from build123d import *

# Parameters (mm, degrees)
SKETCH1_R               = 35
BOSS_EXTRUDE1_DEPTH     = 10
CHAMFER1_SIZE           = 1
CUT_EXTRUDE1_DEPTH      = 11
SKETCH3_R               = 1.5
CUT_EXTRUDE2_DEPTH      = 11
CUT_EXTRUDE3_DEPTH      = 10
SKETCH5_R               = 9.729015648
BOSS_EXTRUDE2_DEPTH     = 3
SKETCH6_R               = 0.75
CUT_EXTRUDE4_DEPTH      = 36
CUT_EXTRUDE4_DEPTH_BACK = 36
CHAMFER2_SIZE           = 3


with BuildPart() as part:
    # Sketch1 → Boss-Extrude1 (new body)
    with BuildSketch(Plane(origin=(0, 0, 0), x_dir=(0, 0, -1), z_dir=(1, 0, 0))):
        Circle(SKETCH1_R)
        with BuildLine():
            Line((-5, 29.580398915), (-5, 8.660254038))
            ThreePointArc((-5, 8.660254038), (0, -10), (5, 8.660254038))
            Line((5, 8.660254038), (5, 29.580398915))
            ThreePointArc((5, 29.580398915), (0, -30), (-5, 29.580398915))
        make_face(mode=Mode.SUBTRACT)
    extrude(amount=BOSS_EXTRUDE1_DEPTH)

    # Chamfer1
    chamfer1_edges = [part.edges().sort_by_distance(p)[0] for p in [
        (0, 0, 35),
        (10, 0, 35),
    ]]
    chamfer(chamfer1_edges, length=CHAMFER1_SIZE)

    # Sketch2 → Cut-Extrude1 (cut, through all)
    with BuildSketch(Plane(origin=(10, 0, 0), x_dir=(0, 0, -1), z_dir=(1, 0, 0))):
        with BuildLine():
            Line((0, 35), (0, 34))
            ThreePointArc((0, 34), (3.553967751, 33.813744443), (7.068997488, 33.257018425))
            Line((7.068997488, 33.257018425), (7.276909179, 34.235166026))
            ThreePointArc((7.276909179, 34.235166026), (3.658496214, 34.808266338), (0, 35))
        make_face()
        with BuildLine():
            Line((15.185930869, 31.533910377), (14.75204713, 30.632941509))
            ThreePointArc((14.75204713, 30.632941509), (17.873248174, 28.923122233), (20.79862617, 26.896415178))
            Line((20.79862617, 26.896415178), (21.410350469, 27.687486213))
            ThreePointArc((21.410350469, 27.687486213), (18.398931943, 29.773802299), (15.185930869, 31.533910377))
        make_face()
        with BuildLine():
            Line((27.364101886, 21.822143065), (26.582270404, 21.198653263))
            ThreePointArc((26.582270404, 21.198653263), (28.652512594, 18.303920947), (30.408831861, 15.208647043))
            Line((30.408831861, 15.208647043), (31.303209268, 15.655960191))
            ThreePointArc((31.303209268, 15.655960191), (29.495233553, 18.842271563), (27.364101886, 21.822143065))
        make_face()
        with BuildLine():
            Line((34.122476926, 7.788232688), (33.147549014, 7.565711755))
            ThreePointArc((33.147549014, 7.565711755), (33.756795496, 4.059403634), (33.996195462, 0.508619839))
            Line((33.996195462, 0.508619839), (34.996083563, 0.523579246))
            ThreePointArc((34.996083563, 0.523579246), (34.749642422, 4.178797859), (34.122476926, 7.788232688))
        make_face()
        with BuildLine():
            Line((34.122476926, -7.788232688), (33.147549014, -7.565711755))
            ThreePointArc((33.147549014, -7.565711755), (32.175131049, -10.989128353), (30.850195615, -14.292145763))
            Line((30.850195615, -14.292145763), (31.75755431, -14.712502991))
            ThreePointArc((31.75755431, -14.712502991), (33.121458433, -11.312338011), (34.122476926, -7.788232688))
        make_face()
        with BuildLine():
            Line((27.364101886, -21.822143065), (26.582270404, -21.198653263))
            ThreePointArc((26.582270404, -21.198653263), (24.220787296, -23.861128698), (21.593936175, -26.262176614))
            Line((21.593936175, -26.262176614), (22.229051944, -27.034593573))
            ThreePointArc((22.229051944, -27.034593573), (24.933163393, -24.562926601), (27.364101886, -21.822143065))
        make_face()
        with BuildLine():
            Line((15.185930869, -31.533910377), (14.75204713, -30.632941509))
            ThreePointArc((14.75204713, -30.632941509), (11.469219571, -32.007139866), (8.060732842, -33.030661302))
            Line((8.060732842, -33.030661302), (8.29781322, -34.00215134))
            ThreePointArc((8.29781322, -34.00215134), (11.806549558, -32.948526333), (15.185930869, -31.533910377))
        make_face()
        with BuildLine():
            Line((0, -35), (0, -34))
            ThreePointArc((0, -34), (-3.553967751, -33.813744443), (-7.068997488, -33.257018425))
            Line((-7.068997488, -33.257018425), (-7.276909179, -34.235166026))
            ThreePointArc((-7.276909179, -34.235166026), (-3.658496214, -34.808266338), (0, -35))
        make_face()
        with BuildLine():
            Line((-15.185930869, -31.533910377), (-14.75204713, -30.632941509))
            ThreePointArc((-14.75204713, -30.632941509), (-17.873248174, -28.923122233), (-20.79862617, -26.896415178))
            Line((-20.79862617, -26.896415178), (-21.410350469, -27.687486213))
            ThreePointArc((-21.410350469, -27.687486213), (-18.398931943, -29.773802299), (-15.185930869, -31.533910377))
        make_face()
        with BuildLine():
            Line((-27.364101886, -21.822143065), (-26.582270404, -21.198653263))
            ThreePointArc((-26.582270404, -21.198653263), (-28.652512594, -18.303920947), (-30.408831861, -15.208647043))
            Line((-30.408831861, -15.208647043), (-31.303209268, -15.655960191))
            ThreePointArc((-31.303209268, -15.655960191), (-29.495233553, -18.842271563), (-27.364101886, -21.822143065))
        make_face()
        with BuildLine():
            Line((-34.122476926, -7.788232688), (-33.147549014, -7.565711755))
            ThreePointArc((-33.147549014, -7.565711755), (-33.756795496, -4.059403634), (-33.996195462, -0.508619839))
            Line((-33.996195462, -0.508619839), (-34.996083563, -0.523579246))
            ThreePointArc((-34.996083563, -0.523579246), (-34.749642422, -4.178797859), (-34.122476926, -7.788232688))
        make_face()
        with BuildLine():
            Line((-34.122476926, 7.788232688), (-33.147549014, 7.565711755))
            ThreePointArc((-33.147549014, 7.565711755), (-32.175131049, 10.989128353), (-30.850195615, 14.292145763))
            Line((-30.850195615, 14.292145763), (-31.75755431, 14.712502991))
            ThreePointArc((-31.75755431, 14.712502991), (-33.121458433, 11.312338011), (-34.122476926, 7.788232688))
        make_face()
        with BuildLine():
            Line((-27.364101886, 21.822143065), (-26.582270404, 21.198653263))
            ThreePointArc((-26.582270404, 21.198653263), (-24.220787296, 23.861128698), (-21.593936175, 26.262176614))
            Line((-21.593936175, 26.262176614), (-22.229051944, 27.034593573))
            ThreePointArc((-22.229051944, 27.034593573), (-24.933163393, 24.562926601), (-27.364101886, 21.822143065))
        make_face()
        with BuildLine():
            Line((-15.185930869, 31.533910377), (-14.75204713, 30.632941509))
            ThreePointArc((-14.75204713, 30.632941509), (-11.469219571, 32.007139866), (-8.060732842, 33.030661302))
            Line((-8.060732842, 33.030661302), (-8.29781322, 34.00215134))
            ThreePointArc((-8.29781322, 34.00215134), (-11.806549558, 32.948526333), (-15.185930869, 31.533910377))
        make_face()
    extrude(amount=-CUT_EXTRUDE1_DEPTH, mode=Mode.SUBTRACT)

    # Sketch3 → Cut-Extrude2 (cut, through all)
    with BuildSketch(Plane.ZY):
        Circle(SKETCH3_R)
    extrude(amount=-CUT_EXTRUDE2_DEPTH, mode=Mode.SUBTRACT)

    # Sketch4 → Cut-Extrude3 (cut)
    with BuildSketch(Plane.ZY):
        with BuildLine():
            Line((-3.865553001, -2.4), (3.865553001, -2.4))
            ThreePointArc((3.865553001, -2.4), (4.55, 0), (3.865553001, 2.4))
            Line((3.865553001, 2.4), (-3.865553001, 2.4))
            ThreePointArc((-3.865553001, 2.4), (-4.55, 0), (-3.865553001, -2.4))
        make_face()
    extrude(amount=-CUT_EXTRUDE3_DEPTH, mode=Mode.SUBTRACT)

    # Sketch5 → Boss-Extrude2 (add)
    with BuildSketch(Plane.ZY):
        Circle(SKETCH5_R)
        with BuildLine():
            Line((-3.865553001, 2.4), (3.865553001, 2.4))
            ThreePointArc((3.865553001, 2.4), (4.568220616, 0), (3.865553001, -2.4))
            Line((3.865553001, -2.4), (-3.865553001, -2.4))
            ThreePointArc((-3.865553001, -2.4), (-4.568220616, 0), (-3.865553001, 2.4))
        make_face(mode=Mode.SUBTRACT)
    extrude(amount=BOSS_EXTRUDE2_DEPTH)

    # Sketch6 → Cut-Extrude4 (cut, two sides)
    with BuildSketch(Plane(origin=(0, 0, 0), x_dir=(1, 0, 0), z_dir=(0, 1, 0))) as cut_extrude4_sk:
        with Locations((-1.5, 0)):
            Circle(SKETCH6_R)
    extrude(amount=CUT_EXTRUDE4_DEPTH, mode=Mode.SUBTRACT)
    extrude(cut_extrude4_sk.sketch, amount=-CUT_EXTRUDE4_DEPTH_BACK, mode=Mode.SUBTRACT)

    # Chamfer2
    chamfer2_edges = [part.edges().sort_by_distance(p)[0] for p in [
        (10, 19.120326477, 5),
        (0, -30, 0),
        (0, 19.120326477, -5),
        (0, 19.120326477, 5),
        (10, -30, 0),
        (10, 19.120326477, -5),
    ]]
    chamfer(chamfer2_edges, length=CHAMFER2_SIZE)


solid = part.part
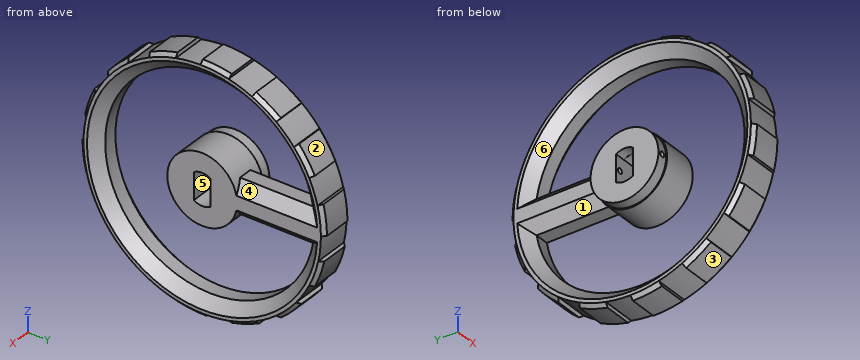
For this review, take the finished solid that the model builds, in its own axes (mm). Face numbers are marked on the shaded views. A direction names the side the tool comes from. Round coordinates to 2 decimals unless told otherwise and drop trailing zeros. One line per question, with ' | ' between items.
Q1. Take a section at A-A (y = 11). State how many separate pieces and enclosed holes the cut face has, and give its area (3 significant figures).
Taken from the geometry:
separate pieces: 3 | enclosed holes: 0 | area: 157 mm²
Q2. For pin 1 (5 mm diameter, centred on x = 3.5, y = 7, fed in from +Z); pin 2 (12 mm diameter, centred on y = 8.5, z = 23, fed in from +X); pin 3 (1.2 mm diameter, centred on x = 4, y = 22.5, fed in from -Z); pin 4 (1.2 mm diameter, centred on x = -1.5, z = 0, fed in from +Y), all flat-tipped, find the tip position at first contact; note any pin that passes through.
Taken from the geometry:
pin 1: stops at z = 34.71 | pin 2: stops at x = 7.52 | pin 3: stops at z = -27.3 | pin 4: passes through
Q3. The part is to be moulded in two halves that separate along Z. For the marked faces 1, 2 and 3, say which applies: released by +Z, released by -Z, zero draft, split by the parting line, or undercut.
Taken from the geometry:
face 1: undercut | face 2: released by +Z | face 3: released by -Z
Q4. Tool access review of the marked faces 4, 5 and 6: name each direction out of +Z, -Z, +X, -X, +Y, -Y from which nothing blocks a thin tool from reaching the whole face with its end or side.
Taken from the geometry:
face 4: +X | face 5: +X, -X | face 6: -X
Q5. For line 1 along X through (y, z) = (6, 0); line 2 along Z through (x, y) = (5, 23); line 3 along Y through (x, z) = (3.25, -2), list the stretches that pass through material, from the lowest coordinate up. Write a range as [from, to].
Taken from the geometry:
line 1: x = [-3, -2.25], [-0.75, 10] | line 2: z = [-26.38, -19.26], [-5, 5], [19.26, 25.04] | line 3: y = [-34.94, -29.93], [-9.8, -2.4], [2.4, 33.94]
